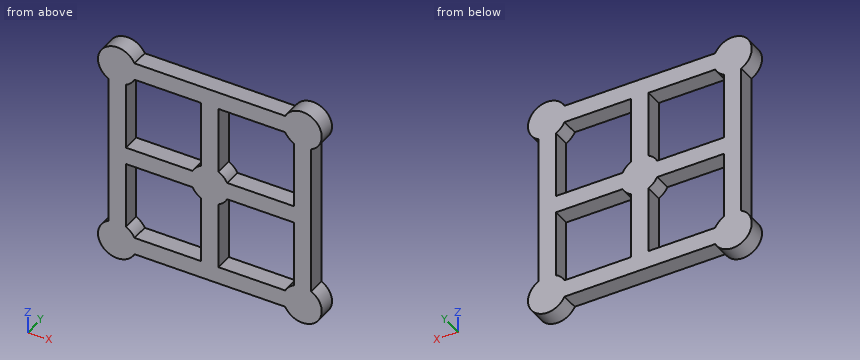
from build123d import *

# Parameters (mm, degrees)
BOSS_EXTRUDE1_DEPTH = 3.556


with BuildPart() as part:
    # Sketch2 → Boss-Extrude1 (new body)
    with BuildSketch(Plane(origin=(0, 0, 0), x_dir=(1, 0, 0), z_dir=(0, 1, 0))):
        with BuildLine():
            Line((15.501804323, -20.828), (-15.501804323, -20.828))
            ThreePointArc((-15.501804323, -20.828), (-21.856330038, -21.856330038), (-20.828, -15.501804323))
            Line((-20.828, -15.501804323), (-20.828, 15.501804323))
            ThreePointArc((-20.828, 15.501804323), (-21.856330038, 21.856330038), (-15.501804323, 20.828))
            Line((-15.501804323, 20.828), (15.501804323, 20.828))
            ThreePointArc((15.501804323, 20.828), (21.856330038, 21.856330038), (20.828, 15.501804323))
            Line((20.828, 15.501804323), (20.828, -15.501804323))
            ThreePointArc((20.828, -15.501804323), (21.856330038, -21.856330038), (15.501804323, -20.828))
        make_face()
        with BuildLine():
            Line((-15.501804323, -17.272), (-1.778, -17.272))
            Line((-1.778, -17.272), (-1.778, -3.548195677))
            ThreePointArc((-1.778, -3.548195677), (-2.806330038, -2.806330038), (-3.548195677, -1.778))
            Line((-3.548195677, -1.778), (-17.272, -1.778))
            Line((-17.272, -1.778), (-17.272, -15.501804323))
            ThreePointArc((-17.272, -15.501804323), (-16.243669962, -16.243669962), (-15.501804323, -17.272))
        make_face(mode=Mode.SUBTRACT)
        with BuildLine():
            Line((-15.501804323, 17.272), (-1.778, 17.272))
            Line((-1.778, 17.272), (-1.778, 3.548195677))
            ThreePointArc((-1.778, 3.548195677), (-2.806330038, 2.806330038), (-3.548195677, 1.778))
            Line((-3.548195677, 1.778), (-17.272, 1.778))
            Line((-17.272, 1.778), (-17.272, 15.501804323))
            ThreePointArc((-17.272, 15.501804323), (-16.243669962, 16.243669962), (-15.501804323, 17.272))
        make_face(mode=Mode.SUBTRACT)
        with BuildLine():
            Line((17.272, -15.501804323), (17.272, -1.778))
            Line((17.272, -1.778), (3.548195677, -1.778))
            ThreePointArc((3.548195677, -1.778), (2.806330038, -2.806330038), (1.778, -3.548195677))
            Line((1.778, -3.548195677), (1.778, -17.272))
            Line((1.778, -17.272), (15.501804323, -17.272))
            ThreePointArc((15.501804323, -17.272), (16.243669962, -16.243669962), (17.272, -15.501804323))
        make_face(mode=Mode.SUBTRACT)
        with BuildLine():
            Line((1.778, 17.272), (1.778, 3.548195677))
            ThreePointArc((1.778, 3.548195677), (2.806330038, 2.806330038), (3.548195677, 1.778))
            Line((3.548195677, 1.778), (17.272, 1.778))
            Line((17.272, 1.778), (17.272, 15.501804323))
            ThreePointArc((17.272, 15.501804323), (16.243669962, 16.243669962), (15.501804323, 17.272))
            Line((15.501804323, 17.272), (1.778, 17.272))
        make_face(mode=Mode.SUBTRACT)
    extrude(amount=BOSS_EXTRUDE1_DEPTH)


solid = part.part
Could you check a few things on this model? Use its own coordinates, in mm. Give positions to 0.01 mm unless a question says otherwise; leave off trailing zeros. Order: outer loops, then holes, each group sorted by start corner. A loop starts at its lowest first (then second) coordinate and runs counter-clockwise, first axis right, second up.
Item 1: If we section it at C-C, the plane z = 14.5: Write out the boundary of the cut face in (x, y).
Item 2: If we section it at D-D, the plane z = -1: Write out the boundary of the cut face in (x, y).
Item 3: I'm going to push flat-ended pins straight in: pin 1 (1.1 mm diameter, centred on x = -11, y = 1.5, fed in from +Z); pin 2 (1.1 mm diameter, centred on y = 2, z = 5, fed in from -X); pin 3 (1.8 mm diameter, centred on x = -13, y = 2, fed in from -Z). Where does each tip first touch, or does it pass through?
Item 4: If we section it at B-B, the plane y = 1.05: Count the separate pieces of the cut face and the enclosed holes in it, plus the area to 3 significant figures.
Item 5: If we section it at A-A, the plane x = 14.5: Write out the boundary of the cut face in (y, z).
Item 6: I need wall thicknesses on line 1 (X direction, y = 1.3, z = -9.5); line 2 (X direction, y = 2.75, z = 21). Which ranges of each line are inside material? Lowest first, please.
Values:
1. outline: (-20.83, 0) - (-17.27, 0) - (-17.27, 3.56) - (-20.83, 3.56) - close; (-1.78, 0) - (1.78, 0) - (1.78, 3.56) - (-1.78, 3.56) - close; (17.27, 0) - (20.83, 0) - (20.83, 3.56) - (17.27, 3.56) - close
2. outline: (-20.83, 0) - (20.83, 0) - (20.83, 3.56) - (-20.83, 3.56) - close
3. pin 1: stops at z = 20.83
3. pin 2: stops at x = -20.83
3. pin 3: stops at z = -20.83
4. separate pieces: 1
4. enclosed holes: 4
4. area: 872 mm2
5. outline: (0, -20.83) - (3.56, -20.83) - (3.56, -17.27) - (0, -17.27) - close; (0, -1.78) - (3.56, -1.78) - (3.56, 1.78) - (0, 1.78) - close; (0, 17.27) - (3.56, 17.27) - (3.56, 20.83) - (0, 20.83) - close
6. line 1: x = -20.83 to -17.27, -1.78 to 1.78, 17.27 to 20.83
6. line 2: x = -22.51 to -15.59, 15.59 to 22.51
